Verification items for the finished model (mm, model axes). A direction names the side the tool comes from. Round coordinates to 2 decimals unless told otherwise and drop trailing zeros. Write each loop counter-clockwise with the first axis right and the second up, starting at its lowest first coordinate (ties: lowest second). Pieces come first, ordered by that corner, then holes. Notation, with made-up numbers: (28.5, -17) - (79.5, -17) arc R12 ccw to (79.5, -3) - close; hole circle Ø10 at (16, 40). An arc over 180 degrees is marked (long way). Answer as a JSON object with one key per item and string values. Group by question number.
1) Set-up check for faces 4 (the cylindrical face through (-50.85, 226.84, 17.23)), 5 (the flat face through (0, -4, 20.52)): record each of +Z, -Z, +X, -X, +Y, -Y from which the full face is reachable in a straight line by a thin tool's end or side.
2) Go/stop test with flat-tipped pins: pin 1 Ø14.5 at (x, y) = (-31, 88) entering from -Z; pin 2 Ø1.6 at (x, y) = (-22, 12.5) entering from -Z; pin 3 Ø12.5 at (y, z) = (12.5, 13.5) entering from +X; pin 4 Ø4 at (y, z) = (198.5, 8) entering from -X. Record where each tip stops, or that it passes through.
3) Section check B-B (y = -27). State how many separate pieces and enclosed holes the cut face has, then the cut area to 3 significant figures.
4) Thickness scan on line 1 (X direction, y = -135, z = 11); line 2 (X direction, y = -122.5, z = 16.25); line 3 (X direction, y = -210, z = 5). Record the ranges inside material, lowest first.
5) Section check A-A (x = -11). Enter the section's corners in (y, z), then the cut area to 3 significant figures.
6) Mould release check, pull along Z, two halves, no side actions. Record for faces 1 (the flat face through (0, -4, 22.52)), 2 (the flat face through (-50.148, -9.387, 5.576)), 3 (the flat face through (21, -4, 13)): +Z half, -Z half, draft (parallel to the pull), parting line (faces both ways), or undercut.
```python
from build123d import *

# Parameters (mm, degrees)
F1_DEPTH       = 250
F2_W           = 38
F2_H           = 13
F3_DEPTH       = 1200
F5_R           = 9
F6_R           = 1
F9_DEPTH       = 500.001
F11_DEPTH      = 23.8214951236
F11_DEPTH_BACK = 526


# Not quite as in the source:
# - an extrude ends at something that could not be found from the text; its depth is read off the source's solid
# - a feature of the source that left no trace in its solid (it failed there, or was rolled back) is left out


with BuildPart() as f1:
    # F0 (on Front) → F1 (new body, symmetric)
    with BuildSketch(Plane.XZ):
        with BuildLine():
            Line((22.5, 62.3204951236), (0, 62.3204951236))
            Line((0, 62.3204951236), (-22.5, 62.3204951236))
            Line((-22.5, 62.3204951236), (-22.5, 63.6204951236))
            Line((-22.5, 63.6204951236), (-45.5824640741, 63.6204951236))
            Line((-45.5824640741, 63.6204951236), (-57.5, 53.6204951236))
            Line((-57.5, 53.6204951236), (-57.5, 49.6204951236))
            Line((-57.5, 49.6204951236), (-40.1794919243, 39.6204951236))
            ThreePointArc((-40.1794919243, 39.6204951236), (0, 43.698039982), (40.1794919243, 39.6204951236))
            Line((40.1794919243, 39.6204951236), (57.5, 49.6204951236))
            Line((57.5, 49.6204951236), (57.5, 53.6204951236))
            Line((57.5, 53.6204951236), (45.5824640741, 63.6204951236))
            Line((45.5824640741, 63.6204951236), (22.5, 63.6204951236))
            Line((22.5, 63.6204951236), (22.5, 62.3204951236))
        make_face()
    extrude(amount=F1_DEPTH, both=True)

    # F2 (on face) → F3 (cut)
    with BuildSketch(Plane.XZ.offset(250)):
        with Locations((0, 53.8204951236)):
            Rectangle(F2_W, F2_H)
    extrude(amount=-F3_DEPTH, mode=Mode.SUBTRACT)

    # F5
    f5_edges = [f1.edges().sort_by_distance(p)[0] for p in [
        (45.582464, 0, 63.620495),
        (40.179492, 0, 39.620495),
        (-40.179492, 0, 39.620495),
        (-45.582464, 0, 63.620495),
    ]]
    fillet(f5_edges, radius=F5_R)

    # F6
    f6_edges = [f1.edges().sort_by_distance(p)[0] for p in [
        (-57.5, 0, 53.620495),
        (-57.5, 0, 49.620495),
        (57.5, 0, 53.620495),
        (57.5, 0, 49.620495),
    ]]
    fillet(f6_edges, radius=F6_R)


with BuildPart() as f1_1:
    # F7: moved
    add(f1.part.moved(Location((0, 0, -39.8))))

    # F8 (on face) → F9 (cut, through all)
    with BuildSketch(Plane.XZ.offset(250)):
        with BuildLine():
            ThreePointArc((22.5, 22.5204951236), (23.2333239744, 23.4636627961), (24.3734993995, 23.8204951236))
            Line((24.3734993995, 23.8204951236), (22.5, 23.8204951236))
            Line((22.5, 23.8204951236), (22.5, 22.5204951236))
        make_face()
        with BuildLine():
            ThreePointArc((-24.3734993995, 23.8204951236), (-23.2333239744, 23.4636627961), (-22.5, 22.5204951236))
            Line((-22.5, 22.5204951236), (-22.5, 23.8204951236))
            Line((-22.5, 23.8204951236), (-24.3734993995, 23.8204951236))
        make_face()
        with BuildLine():
            ThreePointArc((-42.1022690923, 3.2400121158), (-39.7790673433, 2.4018170628), (-37.3093701274, 2.4226251111))
            ThreePointArc((-37.3093701274, 2.4226251111), (-29.1789785809, 3.779472859), (-21, 4.8034903809))
            Line((-21, 4.8034903809), (-21, 20.5204952508))
            Line((-21, 20.5204952508), (-22.5, 20.5204952508))
            ThreePointArc((-22.5, 20.5204952508), (-23.2333240107, 21.4636628361), (-24.3734993995, 21.8204951236))
            Line((-24.3734993995, 21.8204951236), (-42.3067319657, 21.8204951236))
            ThreePointArc((-42.3067319657, 21.8204951236), (-44.7008729689, 21.3983434691), (-46.8062452335, 20.1828062254))
            Line((-46.8062452335, 20.1828062254), (-55.5, 12.8878798072))
            Line((-55.5, 12.8878798072), (-55.5, 10.9751956619))
            Line((-55.5, 10.9751956619), (-42.1022690923, 3.2400121158))
        make_face()
        with BuildLine():
            ThreePointArc((24.3734993995, 21.8204951236), (23.2333240107, 21.4636628361), (22.5, 20.5204952508))
            Line((22.5, 20.5204952508), (21, 20.5204952508))
            Line((21, 20.5204952508), (21, 4.8034903809))
            ThreePointArc((21, 4.8034903809), (29.1789785809, 3.779472859), (37.3093701274, 2.4226251111))
            ThreePointArc((37.3093701274, 2.4226251111), (39.7790673433, 2.4018170628), (42.1022690923, 3.2400121158))
            Line((42.1022690923, 3.2400121158), (55.5, 10.9751956619))
            Line((55.5, 10.9751956619), (55.5, 12.8878798072))
            Line((55.5, 12.8878798072), (46.8062452335, 20.1828062254))
            ThreePointArc((46.8062452335, 20.1828062254), (44.7008729689, 21.3983434691), (42.3067319657, 21.8204951236))
            Line((42.3067319657, 21.8204951236), (24.3734993995, 21.8204951236))
        make_face()
    extrude(amount=-F9_DEPTH, mode=Mode.SUBTRACT)

    # F10 (on Top) → F11 (cut, two sides)
    with BuildSketch(Plane.XY) as f11_sk:
        with BuildLine():
            ThreePointArc((-57.5, 200), (0, 257.5), (57.5, 200))
            Line((57.5, 200), (57.5, 280))
            Line((57.5, 280), (-57.5, 280))
            Line((-57.5, 280), (-57.5, 200))
        make_face()
    extrude(amount=F11_DEPTH, mode=Mode.SUBTRACT)
    extrude(f11_sk.sketch, amount=-F11_DEPTH_BACK, mode=Mode.SUBTRACT)


solid = f1_1.part
```
Returned:
{
 "1": {"face 4": "+Z, -Z, -X, +Y", "face 5": "+Y, -Y"},
 "2": {"pin 1": "z = 0.31", "pin 2": "z = 2.59", "pin 3": "x = 57.5", "pin 4": "x = -57.42"},
 "3": {"separate pieces": "1", "enclosed holes": "3", "area": "622 mm2"},
 "4": {"line 1": "-57.5 to -55.5, -21 to -19, 19 to 21, 55.5 to 57.5", "line 2": "-54.6 to -51.49, -21 to -19, 19 to 21, 51.49 to 54.6", "line 3": "-49.15 to -45.15, -21 to 21, 45.15 to 49.15"},
 "5": {"outline": "(-250, 3.6) - (250, 3.6) - (250, 7.52) - (-250, 7.52) - close; (-250, 20.52) - (250, 20.52) - (250, 22.52) - (-250, 22.52) - close", "area": "2,960 mm2"},
 "6": {"face 1": "+Z half", "face 2": "-Z half", "face 3": "undercut"}
}
